Geometry check sheet. Reference: the model listing, model coordinates, mm. Face numbers are marked on the shaded views. A direction names the side the tool comes from. Round coordinates to 2 decimals unless told otherwise and drop trailing zeros. Write each loop counter-clockwise with the first axis right and the second up, starting at its lowest first coordinate (ties: lowest second). Pieces come first, ordered by that corner, then holes. Notation, with made-up numbers: (-11, -20.75) - (41, -20.75) arc R17 ccw to (41, 12.25) - close; hole circle Ø7 at (39.25, 14.25). An arc over 180 degrees is marked (long way). Return JSON: item names as keys, results as strings.
```python
from build123d import *

# Parameters (mm, degrees)
F0_R     = 25.149299
F1_DEPTH = 88
F2_W     = 88.428743
F2_H     = 40.751
F3_DEPTH = 50
F5_DEPTH = 16
F6_R     = 6.130245
F7_DEPTH = 7.424758


with BuildPart() as f1:
    # F0 (on Top) → F1 (new body)
    with BuildSketch(Plane.XY):
        with BuildLine():
            Line((0, 75.826563), (0, 0))
            Line((0, 0), (47.806516, 0))
            Line((47.806516, 0), (47.806516, 0.408337))
            ThreePointArc((47.806516, 0.408337), (85.31146, 37.913281), (47.806516, 75.418226))
            Line((47.806516, 75.418226), (47.806516, 75.826563))
            Line((47.806516, 75.826563), (0, 75.826563))
        make_face()
        with Locations((47.806516, 37.913281)):
            Circle(F0_R, mode=Mode.SUBTRACT)
    extrude(amount=F1_DEPTH)

    # F2 (on Right) → F3 (join)
    with BuildSketch(Plane.YZ):
        with Locations((-44.214371, 20.3755)):
            Rectangle(F2_W, F2_H)
        with BuildLine():
            ThreePointArc((-18.372269, 33.326242), (-5.31868, 23.097255), (-16.589452, 10.93181))
            Line((-16.589452, 10.93181), (-68.615849, 11.094638))
            ThreePointArc((-68.615849, 11.094638), (-80.794064, 22.111374), (-68.798059, 33.326242))
            Line((-68.798059, 33.326242), (-18.372269, 33.326242))
        make_face(mode=Mode.SUBTRACT)
    extrude(amount=F3_DEPTH)

    # F4 (on Right) → F5 (join)
    with BuildSketch(Plane.YZ):
        Polygon((-88.187516, 41.383404), (0, 41.383404), (0, 88.175647), align=None)
    extrude(amount=F5_DEPTH)

    # F6 (on face) → F7 (cut, through all)
    with BuildSketch(Plane.XY.offset(40.751)):
        with Locations((32.661412, -44.214372)):
            Circle(F6_R)
    extrude(amount=-F7_DEPTH, mode=Mode.SUBTRACT)


solid = f1.part
```
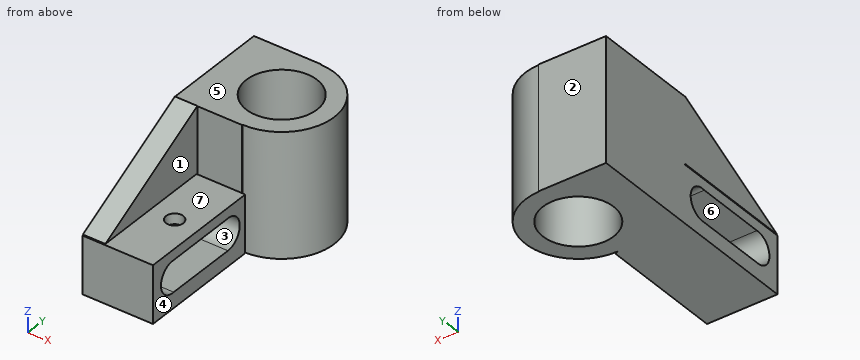
(1) Section check B-B, the plane z = 18. Enter the section's corners in (x, y), plus the area to 3 significant figures.
Response values:
{"outline": "(0, -88.43) - (50, -88.43) - (50, -79.97) - (0, -79.97) - close; (0, -6.1) - (50, -6.1) - (50, 0) - (47.81, 0) - (47.81, 0.41) arc R37.5 ccw to (47.81, 75.42) - (47.81, 75.83) - (0, 75.83) - close; hole circle Ø50.3 at (47.81, 37.91)", "area": "4,580 mm^2"}
(2) Gauge pin test, flat ends, axial feed: pin 1 (1.5 mm diameter, centred on y = -29, z = 37, fed in from -X); pin 2 (8 mm diameter, centred on y = -52.5, z = 47, fed in from +X); pin 3 (20.5 mm diameter, centred on y = -35, z = 19.5, fed in from +X); pin 4 (3 mm diameter, centred on x = 76, z = 33.5, fed in from +Y). Record the tip position at first contact, or that the pin passes through.
Response values:
{"pin 1": "stops at x = 0", "pin 2": "stops at x = 16", "pin 3": "stops at x = 50", "pin 4": "stops at y = 64.26"}
(3) Section check A-A, the plane x = 8. Enter the section's corners in (y, z).
Response values:
{"outline": "(-88.43, 0) - (75.83, 0) - (75.83, 88) - (0, 88) - (0, 88.18) - (-88.19, 41.38) - (0, 41.38) - (0, 40.75) - (-88.43, 40.75) - close; hole (-68.8, 33.33) arc R11.16 ccw (long way) to (-68.62, 11.09) - (-16.59, 10.93) arc R11.27 ccw (long way) to (-18.37, 33.33) - close"}
(4) Access from +Z, -Z, +X, -X, +Y, -Y to the whole of each face (thin tool, end or side, straight path). Record for the marked faces 4, 5, 6 and 7.
Response values:
{"face 4": "+Z, -Z, +X, -Y", "face 5": "+Z, +X, -X, +Y", "face 6": "+X, -X", "face 7": "+X, -X, -Y"}
(5) Section check C-C, the plane y = 53.5. Enter the section's corners in (x, z).
Response values:
{"outline": "(0, 0) - (28.07, 0) - (28.07, 88) - (0, 88) - close; (67.54, 0) - (81.92, 0) - (81.92, 88) - (67.54, 88) - close"}
(6) Material ranges on line 1 along Z through (x, y) = (40.5, -16.5); line 2 along Z through (x, y) = (15, 68); line 3 along X through (y, z) = (50, 33), recorded low to high. Write a range as [from, to].
Response values:
{"line 1": "z = [0, 10.93], [33.47, 40.75]", "line 2": "z = [0, 88]", "line 3": "x = [0, 25.75], [69.86, 83.31]"}
(7) Release check for a two-part mould opening along Y. For the marked faces 1, 2 and 3 record: pulls with the +Y half, pulls with the -Y half, needs draft (parallel to the pull), parting line crosses it, or undercut.
Response values:
{"face 1": "needs draft", "face 2": "pulls with the +Y half", "face 3": "undercut"}
(8) Section check D-D, the plane x = 67. Enter the section's corners in (y, z).
Response values:
{"outline": "(5.69, 0) - (21.66, 0) - (21.66, 88) - (5.69, 88) - close; (54.16, 0) - (70.13, 0) - (70.13, 88) - (54.16, 88) - close"}
